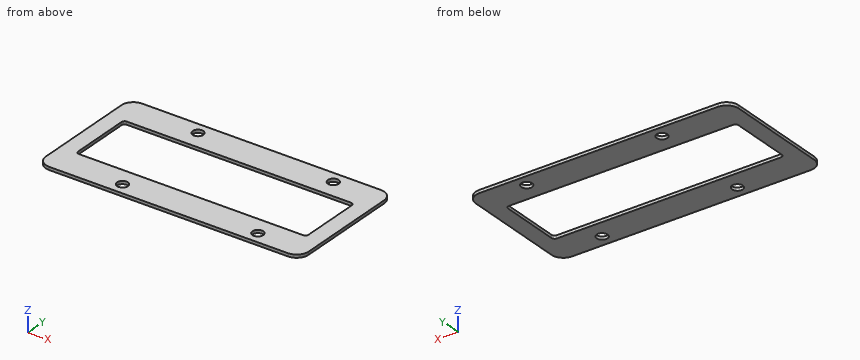
```python
from build123d import *

# Parameters (mm, degrees)
SKETCH_W    = 87.4
SKETCH_H    = 42.4
SKETCH_R    = 1.8
SKETCH_W_2  = 76.6
SKETCH_H_2  = 21.8
PAD_DEPTH   = 1
FILLET_R    = 4
FILLET001_R = 1


with BuildPart() as part:
    # Sketch → Pad (new body)
    with BuildSketch(Plane.XY):
        Rectangle(SKETCH_W, SKETCH_H)
        with Locations((-18.2, 17.2)):
            Circle(SKETCH_R, mode=Mode.SUBTRACT)
        with Locations((-18.2, -17.2)):
            Circle(SKETCH_R, mode=Mode.SUBTRACT)
        with Locations((26.8, -17.2)):
            Circle(SKETCH_R, mode=Mode.SUBTRACT)
        with Locations((26.8, 17.2)):
            Circle(SKETCH_R, mode=Mode.SUBTRACT)
        Rectangle(SKETCH_W_2, SKETCH_H_2, mode=Mode.SUBTRACT)
    extrude(amount=PAD_DEPTH)

    # Fillet
    fillet_edges = [part.edges().sort_by_distance(p)[0] for p in [
        (43.7, -21.2, 0.5),
        (-43.7, -21.2, 0.5),
        (43.7, 21.2, 0.5),
        (-43.7, 21.2, 0.5),
    ]]
    fillet(fillet_edges, radius=FILLET_R)

    # Fillet001
    fillet001_edges = [part.edges().sort_by_distance(p)[0] for p in [
        (38.3, 10.9, 0.5),
        (38.3, -10.9, 0.5),
        (-38.3, -10.9, 0.5),
        (-38.3, 10.9, 0.5),
    ]]
    fillet(fillet001_edges, radius=FILLET001_R)


solid = part.part
```
Model file for the job. Use its own axes, mm. Coordinates: 2 decimals unless noted, no trailing zeros. Order: outer loops, then holes, each group sorted by start corner. A loop starts at its lowest first (then second) coordinate and runs counter-clockwise, first axis right, second up. Notation, with made-up numbers: (33.25, 83.25) -> (39.25, 83.25) arc R10 ccw to (39.25, 93.25) -> close; hole circle Ø4 at (42, 62). An arc over 180 degrees is marked (long way). Answer as a JSON object with one key per item and string values. Group by question number.
1) Drill centre lines: L1, parallel to Y at x = -18.2, z = 0.5; L2, parallel to X at y = 1, z = 0.1; L3, parallel to Y at x = 29, z = 0.65. Where is each one in solid material? Low to high.
2) Cut at C-C, the plane x = -21. Write the cut outline in (y, z).
3) Cut at A-A, the plane y = -7.5. Write the cut outline in (x, z).
4) Flat gauge pin, fed straight in: pin 1 (2 mm diameter, centred on x = 26.8, y = -17.2, fed in from -Z). Where does the tip first touch, or does it go through?
5) Cut at D-D, the plane y = -18. Write the cut outline in (x, z).
6) Cut at B-B, the plane z = 0.6. Write the cut outline in (x, y).
Check values:
{
 "1": {"L1": "y = -21.2 to -19, -15.4 to -10.9, 10.9 to 15.4, 19 to 21.2", "L2": "x = -43.7 to -38.3, 38.3 to 43.7", "L3": "y = -21.2 to -10.9, 10.9 to 21.2"},
 "2": {"outline": "(-21.2, 0) -> (-10.9, 0) -> (-10.9, 1) -> (-21.2, 1) -> close; (10.9, 0) -> (21.2, 0) -> (21.2, 1) -> (10.9, 1) -> close"},
 "3": {"outline": "(-43.7, 0) -> (-38.3, 0) -> (-38.3, 1) -> (-43.7, 1) -> close; (38.3, 0) -> (43.7, 0) -> (43.7, 1) -> (38.3, 1) -> close"},
 "4": {"pin 1": "passes through"},
 "5": {"outline": "(-43.62, 0) -> (-19.81, 0) -> (-19.81, 1) -> (-43.62, 1) -> close; (-16.59, 0) -> (25.19, 0) -> (25.19, 1) -> (-16.59, 1) -> close; (28.41, 0) -> (43.62, 0) -> (43.62, 1) -> (28.41, 1) -> close"},
 "6": {"outline": "(-43.7, -17.2) arc R4 ccw to (-39.7, -21.2) -> (39.7, -21.2) arc R4 ccw to (43.7, -17.2) -> (43.7, 17.2) arc R4 ccw to (39.7, 21.2) -> (-39.7, 21.2) arc R4 ccw to (-43.7, 17.2) -> close; hole (-38.3, -9.9) arc R1 ccw to (-37.3, -10.9) -> (37.3, -10.9) arc R1 ccw to (38.3, -9.9) -> (38.3, 9.9) arc R1 ccw to (37.3, 10.9) -> (-37.3, 10.9) arc R1 ccw to (-38.3, 9.9) -> close; hole circle Ø3.6 at (-18.2, -17.2); hole circle Ø3.6 at (-18.2, 17.2); hole circle Ø3.6 at (26.8, -17.2); hole circle Ø3.6 at (26.8, 17.2)"}
}
